```python
from build123d import *

# Parameters (mm, degrees)
SKETCH_1_W             = 50
SKETCH_1_H             = 50
EXTRUDE_1_DEPTH        = 2
SKETCH_2_R             = 1
CUT_EXTRUDE_1685_DEPTH = 71.738956735
SKETCH_3_R             = 19.75
CUT_EXTRUDE_2158_DEPTH = 1


with BuildPart() as part:
    # Эскиз1 → Бобышка-Вытянуть1 (new body)
    with BuildSketch(Plane(origin=(0, 66.754264805, 0), x_dir=(-1, 0, 0), z_dir=(0, 0, 1))):
        with Locations((25, 41.754264805)):
            Rectangle(SKETCH_1_W, SKETCH_1_H)
    extrude(amount=EXTRUDE_1_DEPTH)

    # Эскиз2 → Cut-Extrude 1685 (cut, through all)
    with BuildSketch(Plane.XY.offset(2)):
        with Locations((-25, 25)):
            Circle(SKETCH_2_R)
        with Locations((-20, 25)):
            Circle(SKETCH_2_R)
        with Locations((-15, 25)):
            Circle(SKETCH_2_R)
        with Locations((-10, 25)):
            Circle(SKETCH_2_R)
        with Locations((-22.5, 20.669872981)):
            Circle(SKETCH_2_R)
        with Locations((-20, 16.339745962)):
            Circle(SKETCH_2_R)
        with Locations((-17.5, 12.009618943)):
            Circle(SKETCH_2_R)
        with Locations((-27.5, 20.669872981)):
            Circle(SKETCH_2_R)
        with Locations((-30, 16.339745962)):
            Circle(SKETCH_2_R)
        with Locations((-32.5, 12.009618943)):
            Circle(SKETCH_2_R)
        with Locations((-30, 25)):
            Circle(SKETCH_2_R)
        with Locations((-35, 25)):
            Circle(SKETCH_2_R)
        with Locations((-40, 25)):
            Circle(SKETCH_2_R)
        with Locations((-27.5, 29.330127019)):
            Circle(SKETCH_2_R)
        with Locations((-30, 33.660254038)):
            Circle(SKETCH_2_R)
        with Locations((-32.5, 37.990381057)):
            Circle(SKETCH_2_R)
        with Locations((-22.5, 29.330127019)):
            Circle(SKETCH_2_R)
        with Locations((-20, 33.660254038)):
            Circle(SKETCH_2_R)
        with Locations((-17.5, 37.990381057)):
            Circle(SKETCH_2_R)
        with Locations((-25, 16.339745962)):
            Circle(SKETCH_2_R)
        with Locations((-27.5, 12.009618943)):
            Circle(SKETCH_2_R)
        with Locations((-22.5, 12.009618943)):
            Circle(SKETCH_2_R)
        with Locations((-32.5, 20.669872981)):
            Circle(SKETCH_2_R)
        with Locations((-37.5, 20.669872981)):
            Circle(SKETCH_2_R)
        with Locations((-35, 16.339745962)):
            Circle(SKETCH_2_R)
        with Locations((-32.5, 29.330127019)):
            Circle(SKETCH_2_R)
        with Locations((-35, 33.660254038)):
            Circle(SKETCH_2_R)
        with Locations((-37.5, 29.330127019)):
            Circle(SKETCH_2_R)
        with Locations((-25, 33.660254038)):
            Circle(SKETCH_2_R)
        with Locations((-22.5, 37.990381057)):
            Circle(SKETCH_2_R)
        with Locations((-27.5, 37.990381057)):
            Circle(SKETCH_2_R)
        with Locations((-17.5, 29.330127019)):
            Circle(SKETCH_2_R)
        with Locations((-12.5, 29.330127019)):
            Circle(SKETCH_2_R)
        with Locations((-15, 33.660254038)):
            Circle(SKETCH_2_R)
        with Locations((-17.5, 20.669872981)):
            Circle(SKETCH_2_R)
        with Locations((-15, 16.339745962)):
            Circle(SKETCH_2_R)
        with Locations((-12.5, 20.669872981)):
            Circle(SKETCH_2_R)
    extrude(amount=-CUT_EXTRUDE_1685_DEPTH, mode=Mode.SUBTRACT)

    # Эскиз3 → Cut-Extrude 2158 (cut)
    with BuildSketch(Plane.XY.offset(2)):
        with Locations((-25, 25)):
            Circle(SKETCH_3_R)
    extrude(amount=-CUT_EXTRUDE_2158_DEPTH, mode=Mode.SUBTRACT)


solid = part.part
```
Geometry: final body of the model. Coordinates: model frame, mm. A direction names the side the tool comes from. Round coordinates to 2 decimals unless told otherwise and drop trailing zeros. Order: outer loops, then holes, each group sorted by start corner. A loop starts at its lowest first (then second) coordinate and runs counter-clockwise, first axis right, second up. Notation, with made-up numbers: (72, 2) - (109, 2) arc R21 ccw to (109, 15) - close; hole circle Ø7 at (2, 20.25). An arc over 180 degrees is marked (long way). Use CSV: the item, a comma, the result in double quotes. Start each with the question number.
Q1. Section query C-C (x = -12.5). Return loops of the section in (y, z), and give its area (3 significant figures).
Q2. Access query for faces 1 (the face through (-26.576, 11.627, 0.507)), 2 (the face through (-29.28, 5.72, 1.51)). Directions: +Z, -Z, +X, -X, +Y, -Y. A direction counts if a zero-diameter tool reaches every point of the face in a straight line with its end or side. Return the directions, or none.
Q3. Material intervals for line 1 along Y through (x, z) = (-30, 0.4); line 2 along Y through (x, z) = (-27.5, 0.75); line 3 along Y through (x, z) = (-37.5, 0.45), sorted ascending. Write a range as from..to.
Q4. Section query A-A (x = -20). Return loops of the section in (y, z), and give its area (3 significant figures).
Q5. First-contact query: pin 1 (2.5 mm diameter, centred on x = -32.5, y = 37.99, fed in from +Z); pin 2 (2.5 mm diameter, centred on x = -22.5, y = 37.99, fed in from -Z). Flat tips, straight axial feed; report the tip coordinate or a pass-through.
Q6. Section query B-B (z = 1.3). Return loops of the section in (x, y), and give its area (3 significant figures).
Q7. Section query D-D (y = 44). Return loops of the section in (x, z), and give its area (3 significant figures).
Q8. Mould query, pull axis X, two halves, no side actions, for faces 3 (the face through (0, 25, 1)), 4 (the face through (-8, 14, 2)), 5 (the face through (-39.076, 24.617, 0.507)), 6 (the face through (-50, 25, 1)). Classes: +X half, -X half, draft (parallel to the pull), parting line (faces both ways), or undercut.
Result set:
1,outline,"(0, 0) - (19.67, 0) - (19.67, 1) - (9.71, 1) - (9.71, 2) - (0, 2) - close; (21.67, 0) - (28.33, 0) - (28.33, 1) - (21.67, 1) - close; (30.33, 0) - (50, 0) - (50, 2) - (40.29, 2) - (40.29, 1) - (30.33, 1) - close"
1,area,"65.4 mm2"
2,face 1,"+Z, -Z"
2,face 2,"+Z"
3,line 1,"y = 0..15.34, 17.34..24, 26..32.66, 34.66..50"
3,line 2,"y = 0..11.01, 13.01..19.67, 21.67..28.33, 30.33..36.99, 38.99..50"
3,line 3,"y = 0..19.67, 21.67..28.33, 30.33..50"
4,outline,"(0, 0) - (15.34, 0) - (15.34, 1) - (5.89, 1) - (5.89, 2) - (0, 2) - close; (17.34, 0) - (24, 0) - (24, 1) - (17.34, 1) - close; (26, 0) - (32.66, 0) - (32.66, 1) - (26, 1) - close; (34.66, 0) - (50, 0) - (50, 2) - (44.11, 2) - (44.11, 1) - (34.66, 1) - close"
4,area,"55.8 mm2"
5,pin 1,"stops at z = 1"
5,pin 2,"stops at z = 0"
6,outline,"(-50, 0) - (0, 0) - (0, 50) - (-50, 50) - close; hole circle Ø39.5 at (-25, 25)"
6,area,"1,270 mm2"
7,outline,"(-50, 0) - (0, 0) - (0, 2) - (-19.61, 2) - (-19.61, 1) - (-30.39, 1) - (-30.39, 2) - (-50, 2) - close"
7,area,"89.2 mm2"
8,face 3,"+X half"
8,face 4,"draft"
8,face 5,"undercut"
8,face 6,"-X half"
